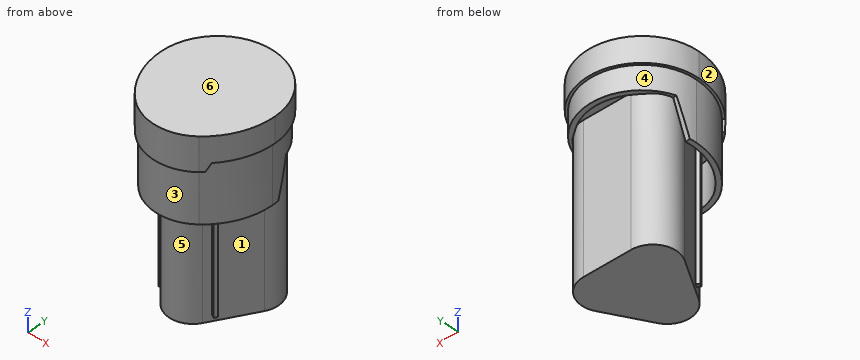
```python
from build123d import *
from OCP.BRepFilletAPI import BRepFilletAPI_MakeChamfer

# Parameters (mm, degrees)
BOSS_EXTRU_1_DEPTH      = 80
BOSS_EXTRU_2_DEPTH      = 10.6
BOSS_EXTRU_3_DEPTH      = 10
BOSS_EXTRU_4_DEPTH      = 3.5
CHANFREIN1_SIZE         = 2
CHANFREIN1_SIZE_2       = 3.5
BOSS_EXTRU_5_DEPTH      = 14.9
CHANFREIN2_SIZE         = 5
CHANFREIN2_SIZE_2       = 14.9
ENL_V_MAT_EXTRU_1_DEPTH = 61.9
BOSS_EXTRU_8_REACH      = 92.636
BOSS_EXTRU_8_START      = -2.5


with BuildPart() as part:
    # Esquisse1 → Boss.-Extru.1 (new body)
    with BuildSketch(Plane.XY):
        with BuildLine():
            Line((-9.999999999999973, 15.773502691896244), (9.999999999999973, 15.773502691896244))
            ThreePointArc((9.999999999999973, 15.773502691896244), (18.66025403784436, 10.773502691896228), (18.66025403784438, 0.7735026918962024))
            Line((18.66025403784438, 0.7735026918962024), (8.660254037844393, -16.54700538379251))
            ThreePointArc((8.660254037844393, -16.54700538379251), (-4.87e-15, -21.5470053837925), (-8.660254037844393, -16.54700538379251))
            Line((-8.660254037844393, -16.54700538379251), (-18.66025403784438, 0.7735026918962024))
            ThreePointArc((-18.66025403784438, 0.7735026918962024), (-18.66025403784441, 10.773502691896235), (-9.999999999999973, 15.773502691896244))
        make_face()
    extrude(amount=BOSS_EXTRU_1_DEPTH)

    # Esquisse2 → Boss.-Extru.2 (add)
    with BuildSketch(Plane.XY.offset(80)):
        with BuildLine():
            Line((0, 23.773502691896258), (0, -28.226497308103742))
            ThreePointArc((0, -28.226497308103742), (-7.138520611844601, -26.935621886911633), (-13.372879499304581, -23.22649730810374))
            ThreePointArc((-13.372879499304581, -23.22649730810374), (-21.14415675858487, -12.819312855059437), (-23.89999999999999, -0.12649730810374363))
            ThreePointArc((-23.89999999999999, -0.12649730810374363), (-16.89985207035848, 16.773354762254744), (0, 23.773502691896258))
        make_face()
    boss_extru_2 = extrude(amount=-BOSS_EXTRU_2_DEPTH)

    # Symétrie1: Boss.-Extru.2 across plane
    add(boss_extru_2.mirror(Plane(origin=(0, 0, 0), x_dir=(0, 0, 1), z_dir=(1, 0, 0))))

    # Esquisse4 → Boss.-Extru.3 (add)
    with BuildSketch(Plane(origin=(0, 0, 69.4), x_dir=(-1, 0, 0), z_dir=(0, 0, -1))):
        with BuildLine():
            ThreePointArc((-12.716812029717252, -22.471795065262707), (-2.04e-15, -27.226497308103735), (12.71681202971725, -22.4717950652627))
            ThreePointArc((12.71681202971725, -22.4717950652627), (20.2341931687673, -12.404624700892555), (22.899999999999995, -0.12649730810373652))
            ThreePointArc((22.899999999999995, -0.12649730810373652), (-6.91e-15, 22.773502691896258), (-22.899999999999995, -0.12649730810373735))
            ThreePointArc((-22.899999999999995, -0.12649730810373735), (-20.234193168767305, -12.404624700892553), (-12.716812029717252, -22.471795065262707))
        make_face()
    extrude(amount=BOSS_EXTRU_3_DEPTH)

    # Esquisse6 → Boss.-Extru.4 (add)
    with BuildSketch(Plane(origin=(0, 0, 69.4), x_dir=(-1, 0, 0), z_dir=(0, 0, -1))):
        with BuildLine():
            Line((14.75, -21.95321690393977), (0, -13.476497308103742))
            Line((0, -13.476497308103742), (0, -28.226497308103742))
            ThreePointArc((0, -28.226497308103742), (7.138520611844594, -26.935621886911633), (13.372879499304576, -23.226497308103735))
            ThreePointArc((13.372879499304576, -23.226497308103735), (14.071194795630928, -22.600407707254973), (14.75, -21.95321690393977))
        make_face()
    boss_extru_4 = extrude(amount=BOSS_EXTRU_4_DEPTH)

    # Symétrie2: Boss.-Extru.4 across plane
    add(boss_extru_4.mirror(Plane(origin=(0, 0, 0), x_dir=(0, 0, 1), z_dir=(1, 0, 0))))

    # Chanfrein1
    chanfrein1_edges_1 = [part.edges().sort_by_distance(p)[0] for p in [
        (-14.299309891443901, -21.69420851920438, 69.4),
    ]]
    chanfrein1_side_1 = [part.faces().sort_by_distance(p)[0] for p in [
        (-14.319240730556658, -21.659527664943543, 69.4),
    ]]
    chanfrein1_edges_2 = [part.edges().sort_by_distance(p)[0] for p in [
        (14.299309891443906, -21.694208519204384, 69.4),
    ]]
    chanfrein1_side_2 = [part.faces().sort_by_distance(p)[0] for p in [
        (14.319240730556663, -21.659527664943546, 69.4),
    ]]
    chanfrein1 = BRepFilletAPI_MakeChamfer(part.part.solid().wrapped)
    for e in chanfrein1_edges_1:
        chanfrein1.Add(CHANFREIN1_SIZE - 0.0001, CHANFREIN1_SIZE_2 - 0.0001, e.wrapped, chanfrein1_side_1[0].wrapped)
    for e in chanfrein1_edges_2:
        chanfrein1.Add(CHANFREIN1_SIZE - 0.0001, CHANFREIN1_SIZE_2 - 0.0001, e.wrapped, chanfrein1_side_2[0].wrapped)
    add(Compound.cast(chanfrein1.Shape()), mode=Mode.REPLACE)  # a hair under: the kernel refuses the full size

    # Esquisse7 → Boss.-Extru.5 (add)
    with BuildSketch(Plane(origin=(0, 0, 59.4), x_dir=(-1, 0, 0), z_dir=(0, 0, -1))):
        with BuildLine():
            Line((-6.79e-15, -27.22649730810374), (0, 0))
            Line((0, 0), (22.71563338320109, 2.7735026918962267))
            ThreePointArc((22.71563338320109, 2.7735026918962267), (22.853861867037974, 1.3264299999015228), (22.899999999999995, -0.12649730810374016))
            ThreePointArc((22.899999999999995, -0.12649730810374016), (20.2341931687673, -12.404624700892562), (12.716812029717245, -22.471795065262707))
            ThreePointArc((12.716812029717245, -22.471795065262707), (6.788307992740876, -25.998951656029643), (-6.79e-15, -27.22649730810374))
        make_face()
    boss_extru_5 = extrude(amount=BOSS_EXTRU_5_DEPTH)

    # Symétrie4: Boss.-Extru.5 across plane
    add(boss_extru_5.mirror(Plane(origin=(0, 0, 0), x_dir=(0, 0, 1), z_dir=(1, 0, 0))))

    # Chanfrein2
    chanfrein2_edges_1 = [part.edges().sort_by_distance(p)[0] for p in [
        (21.059128460282075, 2.5712489935136453, 59.4),
    ]]
    chanfrein2_side_1 = [part.faces().sort_by_distance(p)[0] for p in [
        (21.04700879877706, 2.6705118456034573, 59.4),
    ]]
    chanfrein2_edges_2 = [part.edges().sort_by_distance(p)[0] for p in [
        (-21.059128460282082, 2.571248993513646, 59.4),
    ]]
    chanfrein2_side_2 = [part.faces().sort_by_distance(p)[0] for p in [
        (-21.059128460282082, 2.571248993513646, 59.3),
    ]]
    chanfrein2 = BRepFilletAPI_MakeChamfer(part.part.solid().wrapped)
    for e in chanfrein2_edges_1:
        chanfrein2.Add(CHANFREIN2_SIZE - 0.0001, CHANFREIN2_SIZE_2 - 0.0001, e.wrapped, chanfrein2_side_1[0].wrapped)
    for e in chanfrein2_edges_2:
        chanfrein2.Add(CHANFREIN2_SIZE_2 - 0.0001, CHANFREIN2_SIZE - 0.0001, e.wrapped, chanfrein2_side_2[0].wrapped)
    add(Compound.cast(chanfrein2.Shape()), mode=Mode.REPLACE)  # a hair under: the kernel refuses the full size

    # Esquisse8 → Enlèv. mat.-Extru.1 (cut)
    with BuildSketch(Plane(origin=(0, 0, 0), x_dir=(-1, 0, 0), z_dir=(0, 0, -1))):
        with BuildLine():
            Line((-20.73173527113113, 2.5202275827259273), (-20.108299540895768, 7.138156637600371))
            ThreePointArc((-20.108299540895768, 7.138156637600371), (-18.785258977060302, 10.95609130242486), (-16.08354229758742, 13.96071913666333))
            Line((-16.08354229758742, 13.96071913666333), (-12.465297452899778, 16.64926972087978))
            ThreePointArc((-12.465297452899778, 16.64926972087978), (8.34e-15, 20.773502691896244), (12.465297452899788, 16.649269720879765))
            Line((12.465297452899788, 16.649269720879765), (16.083542297587456, 13.96071913666329))
            ThreePointArc((16.083542297587456, 13.96071913666329), (18.78525897706036, 10.956091302424788), (20.108299540895814, 7.13815663760026))
            Line((20.108299540895814, 7.13815663760026), (20.73173527113112, 2.5202275827259264))
            ThreePointArc((20.73173527113112, 2.5202275827259264), (20.857891398301028, 1.1995367852285772), (20.89999999999999, -0.12649730810373677))
            ThreePointArc((20.89999999999999, -0.12649730810373677), (18.414265989132176, -11.5752483925588), (11.404677090542576, -20.962390579580656))
            ThreePointArc((11.404677090542576, -20.962390579580656), (1.69e-15, -25.226497308103735), (-11.40467709054258, -20.962390579580664))
            ThreePointArc((-11.40467709054258, -20.962390579580664), (-18.414265989132176, -11.575248392558798), (-20.89999999999999, -0.1264973081037376))
            ThreePointArc((-20.89999999999999, -0.1264973081037376), (-20.85789139830103, 1.1995367852285768), (-20.73173527113113, 2.5202275827259273))
        make_face()
        with BuildLine():
            Line((-18.66025403784436, 0.773502691896218), (-8.660254037844393, -16.54700538379251))
            ThreePointArc((-8.660254037844393, -16.54700538379251), (6.09e-15, -21.547005383792524), (8.660254037844393, -16.54700538379251))
            Line((8.660254037844393, -16.54700538379251), (18.66025403784438, 0.7735026918962024))
            ThreePointArc((18.66025403784438, 0.7735026918962024), (18.66025403784438, 10.773502691896217), (9.999999999999973, 15.773502691896226))
            Line((9.999999999999973, 15.773502691896226), (-9.999999999999973, 15.773502691896244))
            ThreePointArc((-9.999999999999973, 15.773502691896244), (-18.660254037844357, 10.77350269189623), (-18.66025403784436, 0.773502691896218))
        make_face(mode=Mode.SUBTRACT)
    extrude(amount=-ENL_V_MAT_EXTRU_1_DEPTH, mode=Mode.SUBTRACT)

    # Esquisse9 → Boss.-Extru.8 (add, up to next)
    with BuildSketch(Plane(origin=(0, 0, 0), x_dir=(-1, 0, 0), z_dir=(0, 0, -1)).offset(BOSS_EXTRU_8_START), mode=Mode.PRIVATE) as boss_extru_8_sk1:
        Polygon((-10.214359353944898, -13.855216015993522), (-11.599999999999998, -14.655216015993522), (-12.3, -13.442780450695311), (-10.914359353944906, -12.642780450695314), align=None)
    boss_extru_8_tool1 = extrude(boss_extru_8_sk1.sketch, amount=-BOSS_EXTRU_8_REACH, mode=Mode.PRIVATE) - part.part
    # Esquisse9 → Boss.-Extru.8 (add, up to next)
    with BuildSketch(Plane(origin=(0, 0, 0), x_dir=(-1, 0, 0), z_dir=(0, 0, -1)).offset(BOSS_EXTRU_8_START), mode=Mode.PRIVATE) as boss_extru_8_sk2:
        Polygon((10.914359353944906, -12.642780450695314), (10.214359353944898, -13.855216015993522), (11.599999999999998, -14.655216015993522), (12.3, -13.442780450695311), align=None)
    boss_extru_8_tool2 = extrude(boss_extru_8_sk2.sketch, amount=-BOSS_EXTRU_8_REACH, mode=Mode.PRIVATE) - part.part
    add(boss_extru_8_tool1.solids().sort_by_distance((11.25718, -13.648998, 2.5))[0])
    add(boss_extru_8_tool2.solids().sort_by_distance((-11.25718, -13.648998, 2.5))[0])


solid = part.part
```
For this review, take the finished solid that the model builds, in its own axes (mm). Face numbers are marked on the shaded views. A direction names the side the tool comes from. Round coordinates to 2 decimals unless told otherwise and drop trailing zeros. Write each loop counter-clockwise with the first axis right and the second up, starting at its lowest first coordinate (ties: lowest second). Pieces come first, ordered by that corner, then holes.
1) Take a section at D-D on z = 16. Give the boundary of the cut face in (x, y).
Answer below:
outline: (-18.66, 0.77) - (-10.91, -12.64) - (-12.3, -13.44) - (-11.6, -14.66) - (-10.21, -13.86) - (-8.66, -16.55) arc R10 ccw to (8.66, -16.55) - (10.21, -13.86) - (11.6, -14.66) - (12.3, -13.44) - (10.91, -12.64) - (18.66, 0.77) arc R10 ccw to (10, 15.77) - (-10, 15.77) arc R10 ccw to start
2) Insertion check: pin 1 Ø2 at (x, y) = (-11.5, -14) entering from -Z; pin 2 Ø22 at (x, y) = (5, -5.5) entering from -Z; pin 3 Ø1.5 at (x, z) = (18, 52) entering from +Y; pin 4 Ø1 at (x, z) = (4.5, 69.5) entering from -Y. Each pin has a flat end and moves straight along its axis. Give the tip position at first contact, or say it passes through.
Answer below:
pin 1: stops at z = 2.5
pin 2: stops at z = 0
pin 3: stops at y = 12.66
pin 4: stops at y = -27.83
3) For line 1 along X through (y, z) = (-16, 58); line 2 along X through (y, z) = (-14.5, 50); line 3 along Z through (x, y) = (2, 16), list the stretches that pass through material, from the lowest coordinate up.
Answer below:
line 1: x = -18.29 to -15.88, -8.98 to 8.98, 15.88 to 18.29
line 2: x = -19.18 to -16.86, -11.69 to -11.33, -9.84 to 9.84, 11.33 to 11.69, 16.86 to 19.18
line 3: z = 61.9 to 80
4) Machinability: for the marked faces 1 and 2, which of the approach directions +Z, -Z, +X, -X, +Y, -Y give a long, thin tool a straight path to every point of the face, cutting with its end or side? Answer none if there is none.
Answer below:
face 1: -Z
face 2: +Z, -Z, -X, -Y
5) Take a section at C-C on y = 10. Give the boundary of the cut face in (x, z).
Answer below:
outline: (-21.65, 69.4) - (-20.54, 69.4) - (-20.54, 59.4) - (-19.28, 59.4) - (-19.28, 61.9) - (-19.06, 61.9) - (-19.06, 0) - (19.06, 0) - (19.06, 61.9) - (19.28, 61.9) - (19.28, 59.4) - (20.54, 59.4) - (20.54, 69.4) - (21.65, 69.4) - (21.65, 80) - (-21.65, 80) - close
6) Mouldability with a two-part tool opening along Y and no side actions: class the marked faces 3, 4, 5 and 6 as +Y half, -Y half, draft (parallel to the pull), parting line (faces both ways), or undercut.
Answer below:
face 3: -Y half
face 4: +Y half
face 5: undercut
face 6: draft
7) Take a section at B-B on x = 0. Give the boundary of the cut face in (y, z), then the cut area to 3 significant figures.
Answer below:
outline: (-28.23, 65.9) - (-27.23, 65.9) - (-27.23, 44.5) - (-25.23, 44.5) - (-25.23, 61.9) - (-21.55, 61.9) - (-21.55, 0) - (15.77, 0) - (15.77, 61.9) - (20.77, 61.9) - (20.77, 59.4) - (22.77, 59.4) - (22.77, 69.4) - (23.77, 69.4) - (23.77, 80) - (-28.23, 80) - close
area: 3,280 mm2
8) Take a section at A-A on z = 48. Give the boundary of the cut face in (x, y), then the cut area to 3 significant figures.
Answer below:
outline: (-22.9, -0.13) arc R29.61 ccw to (-12.72, -22.47) arc R19.38 ccw to (12.72, -22.47) arc R29.61 ccw to (22.9, -0.13) arc R22.9 ccw to (22.54, 3.93) - (20.57, 3.7) - (20.73, 2.52) arc R20.9 cw to (20.9, -0.13) arc R27.61 cw to (11.4, -20.96) arc R17.38 cw to (-11.4, -20.96) arc R27.61 cw to (-20.9, -0.13) arc R20.9 cw to (-20.73, 2.52) - (-20.57, 3.7) - (-22.54, 3.93) arc R22.9 ccw to start; (-18.66, 0.77) - (-10.91, -12.64) - (-12.3, -13.44) - (-11.6, -14.66) - (-10.21, -13.86) - (-8.66, -16.55) arc R10 ccw to (8.66, -16.55) - (10.21, -13.86) - (11.6, -14.66) - (12.3, -13.44) - (10.91, -12.64) - (18.66, 0.77) arc R10 ccw to (10, 15.77) - (-10, 15.77) arc R10 ccw to start
area: 1,260 mm2
